Geometry check sheet. Reference: drawing and pictorial views, mm from the part's lowest x, y, z. A direction names the side the tool comes from. Give positions to 0.01 mm unless a question says otherwise; leave off trailing zeros. Loops run counter-clockwise (first coordinate to the right, second up) from the corner with the lowest first, then second, coordinate; pieces in that order, holes last. Notation, with made-up numbers: (-30, 14.25) - (0, 14.25) arc R13 ccw to (0, 35.25) - close; hole circle Ø8 at (-12.75, 66). An arc over 180 degrees is marked (long way). Put each result on its own line as item: value. Start each with the question number.
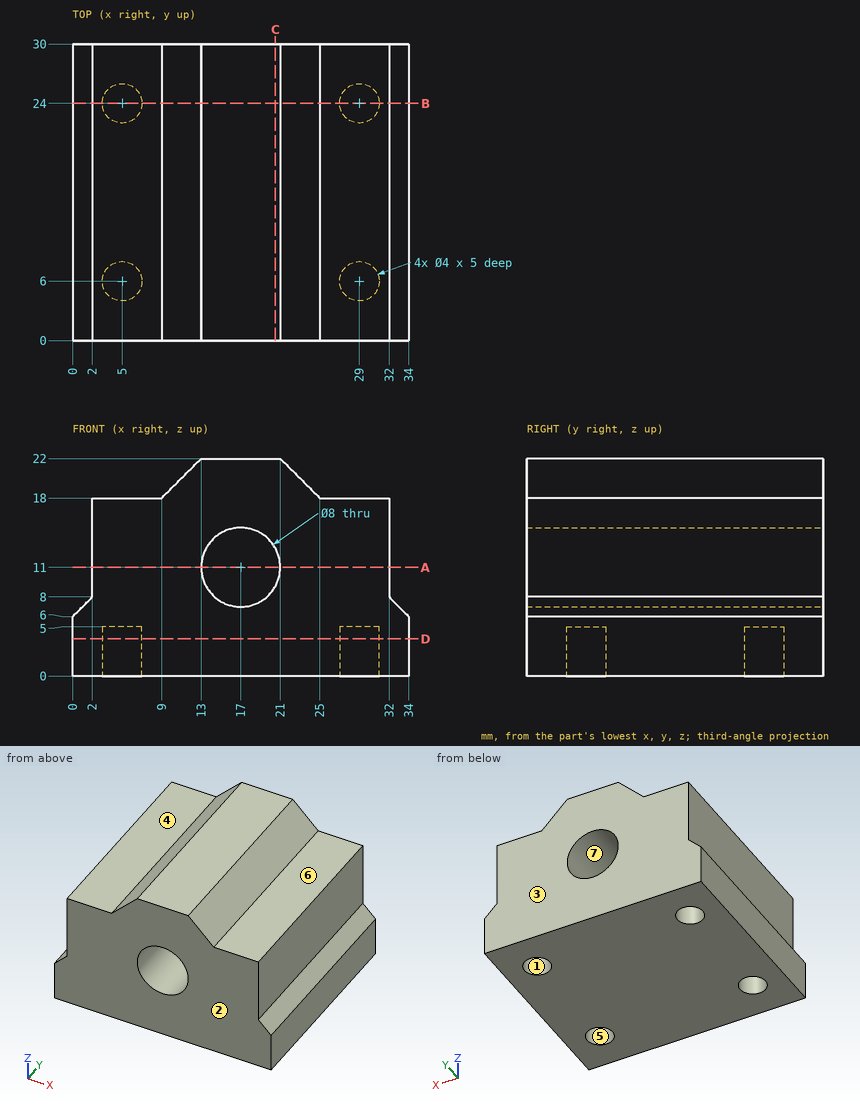
1) Set-up check for the marked faces 4, 5, 6 and 7: record each of +Z, -Z, +X, -X, +Y, -Y from which the full face is reachable in a straight line by a thin tool's end or side.
2) Scan lines: line 1 along Y through (x, z) = (5, 2.25); line 2 along X through (y, z) = (6, 3.9); line 3 along X through (y, z) = (12.25, 11.25). Record each from-to range of solid material in increasing order. Write a range as from..to.
3) Section check D-D, the plane z = 3.75. Enter the section's corners in (x, y), plus the area to 3 significant figures.
4) Depth check by flat-ended pin: P1, Ø1.2, axis at x = 29, y = 6.5, coming from the -Z side; P2, Ø3, axis at x = 30, y = 4.5, coming from the +Z side; P3, Ø3, axis at y = 21, z = 13, coming from the +X side; P4, Ø5, axis at x = 17, z = 11, coming from the -Y side. Enter the tip coordinate at first touch or a pass-through.
5) Section check B-B, the plane y = 24. Enter the section's corners in (x, z), plus the area to 3 significant figures.
6) Section check A-A, the plane z = 11. Enter the section's corners in (x, y).
7) Section check C-C, the plane x = 20.5. Enter the section's corners in (y, z).
8) Draft check along Y on the marked faces 1, 2 and 3. Enter one of: pulls with the +Y half, pulls with the -Y half, needs draft (parallel to the pull), parting line crosses it, or undercut.
Results are:
1. face 4: +Z, -X, +Y, -Y
1. face 5: -Z
1. face 6: +Z, +X, +Y, -Y
1. face 7: +Y, -Y
2. line 1: y = 0..4, 8..22, 26..30
2. line 2: x = 0..3, 7..27, 31..34
2. line 3: x = 2..13.01, 20.99..32
3. outline: (0, 0) - (34, 0) - (34, 30) - (0, 30) - close; hole circle Ø4 at (5, 6); hole circle Ø4 at (5, 24); hole circle Ø4 at (29, 6); hole circle Ø4 at (29, 24)
3. area: 970 mm2
4. P1: stops at z = 5
4. P2: stops at z = 18
4. P3: stops at x = 32
4. P4: passes through
5. outline: (0, 0) - (3, 0) - (3, 5) - (7, 5) - (7, 0) - (27, 0) - (27, 5) - (31, 5) - (31, 0) - (34, 0) - (34, 6) - (32, 8) - (32, 18) - (25, 18) - (21, 22) - (13, 22) - (9, 18) - (2, 18) - (2, 8) - (0, 6) - close; hole circle Ø8 at (17, 11)
5. area: 526 mm2
6. outline: (2, 0) - (13, 0) - (13, 30) - (2, 30) - close; (21, 0) - (32, 0) - (32, 30) - (21, 30) - close
7. outline: (0, 0) - (30, 0) - (30, 9.06) - (0, 9.06) - close; (0, 12.94) - (30, 12.94) - (30, 22) - (0, 22) - close
8. face 1: undercut
8. face 2: pulls with the -Y half
8. face 3: pulls with the +Y half
